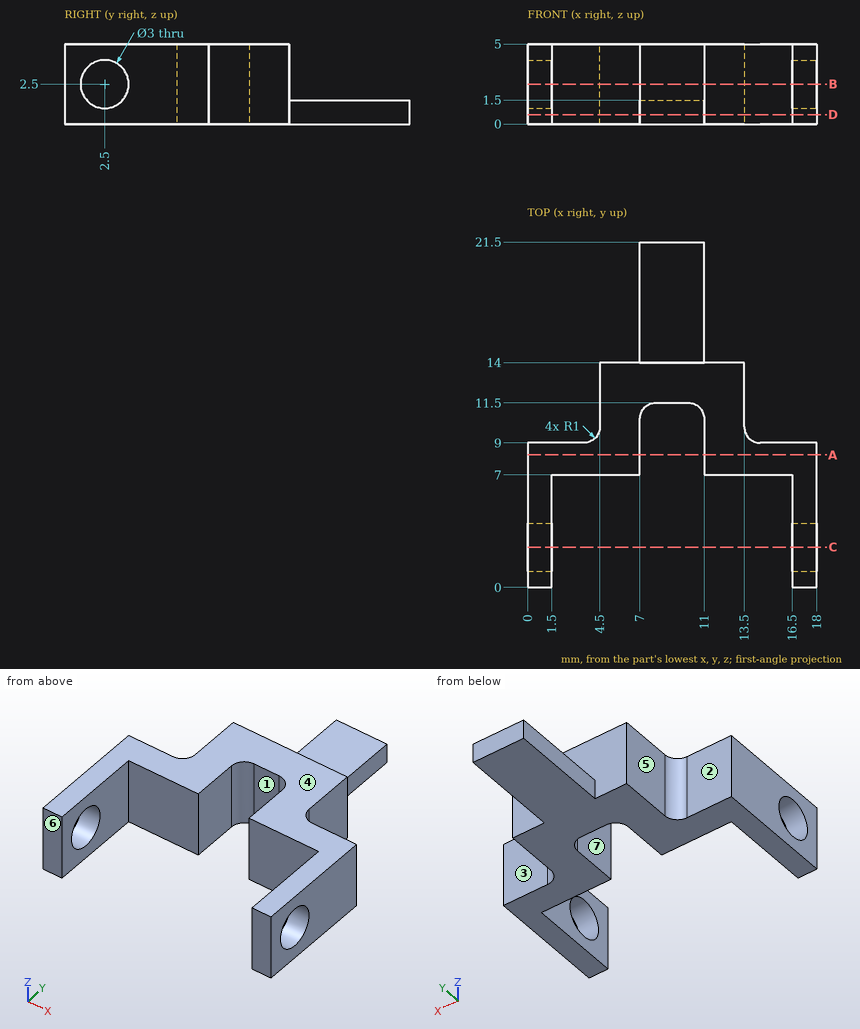
Here's the drawing with two shaded views (mm, measured from the low corner). I have some questions. A direction names the side the tool comes from. Give positions to 0.01 mm unless a question says otherwise; leave off trailing zeros. Order: outer loops, then holes, each group sorted by start corner. A loop starts at its lowest first (then second) coordinate and runs counter-clockwise, first axis right, second up. Notation, with made-up numbers: (86, 83) - (130, 83) arc R33 cw to (130, 113) - close; hole circle Ø9 at (39, -2.75). An arc over 180 degrees is marked (long way). Write each question's results on one line, items separated by ' | '.
1) I'm going to push flat-ended pins straight in: pin 1 Ø1 at (x, z) = (5.5, 4.5) entering from +Y; pin 2 Ø2 at (x, y) = (9.5, 19) entering from +Z; pin 3 Ø1.8 at (y, z) = (8.5, 2) entering from -X; pin 4 Ø4 at (x, y) = (13.5, 2.5) entering from -Z. Where does each tip first touch, or does it pass through?
Final values:
pin 1: stops at y = 14 | pin 2: stops at z = 1.5 | pin 3: stops at x = 0 | pin 4: passes through
2) Suppose I cut it at C-C, the plane y = 2.5. Write out the boundary of the cut face in (x, z), then the cut area to 3 significant figures.
Final values:
outline: (0, 0) - (1.5, 0) - (1.5, 1) - (0, 1) - close; (0, 4) - (1.5, 4) - (1.5, 5) - (0, 5) - close; (16.5, 0) - (18, 0) - (18, 1) - (16.5, 1) - close; (16.5, 4) - (18, 4) - (18, 5) - (16.5, 5) - close | area: 6.00 mm^2
3) Suppose I cut it at B-B, the plane z = 2.5. Write out the boundary of the cut face in (x, y), then the cut area to 3 significant figures.
Final values:
outline: (0, 0) - (1.5, 0) - (1.5, 1) - (0, 1) - close; (0, 4) - (1.5, 4) - (1.5, 7) - (7, 7) - (7, 10.5) arc R1 cw to (8, 11.5) - (10, 11.5) arc R1 cw to (11, 10.5) - (11, 7) - (16.5, 7) - (16.5, 4) - (18, 4) - (18, 9) - (14.5, 9) arc R1 cw to (13.5, 10) - (13.5, 14) - (4.5, 14) - (4.5, 10) arc R1 cw to (3.5, 9) - (0, 9) - close; (16.5, 0) - (18, 0) - (18, 1) - (16.5, 1) - close | area: 75.9 mm^2
4) Suppose I cut it at A-A, the plane y = 8.25. Write out the boundary of the cut face in (x, z), then the cut area to 3 significant figures.
Final values:
outline: (0, 0) - (7, 0) - (7, 5) - (0, 5) - close; (11, 0) - (18, 0) - (18, 5) - (11, 5) - close | area: 70.0 mm^2
5) On a 3-axis mill with a long thin cutter (end or side, diameter ignored), from which of +Z, -Z, +X, -X, +Y, -Y can I reach the whole of each face in a straight line? I mean the marked faces 1, 2, 3 and 4. Say none if no direction works.
Final values:
face 1: +Z, -Z, -Y | face 2: +Z, -Z, -X, +Y | face 3: +Z, -Z, +X, +Y | face 4: +Z, +X, -X, +Y, -Y
6) If we mould it in two halves opening along X, with no side actions, what happens to the marked faces 5, 6 and 7? For each: pulls with the +X half, pulls with the -X half, needs draft (parallel to the pull), parting line crosses it, or undercut.
Final values:
face 5: pulls with the -X half | face 6: needs draft | face 7: undercut
7) Please list where these lines run through material, in increasing order: line 1 along Z through (x, y) = (17.75, 2.5); line 2 along X through (y, z) = (10.5, 0.85); line 3 along X through (y, z) = (1.75, 4.1). Write a range as [from, to].
Final values:
line 1: z = [0, 1], [4, 5] | line 2: x = [4.5, 7], [11, 13.5] | line 3: x = [0, 1.5], [16.5, 18]
8) Suppose I cut it at D-D, the plane z = 0.6. Write out the boundary of the cut face in (x, y), then the cut area to 3 significant figures.
Final values:
outline: (0, 0) - (1.5, 0) - (1.5, 7) - (7, 7) - (7, 10.5) arc R1 cw to (8, 11.5) - (10, 11.5) arc R1 cw to (11, 10.5) - (11, 7) - (16.5, 7) - (16.5, 0) - (18, 0) - (18, 9) - (14.5, 9) arc R1 cw to (13.5, 10) - (13.5, 14) - (11, 14) - (11, 21.5) - (7, 21.5) - (7, 14) - (4.5, 14) - (4.5, 10) arc R1 cw to (3.5, 9) - (0, 9) - close | area: 115 mm^2
